Model file for the job. Use its own axes, mm. Round coordinates to 2 decimals unless told otherwise and drop trailing zeros. Order: outer loops, then holes, each group sorted by start corner. A loop starts at its lowest first (then second) coordinate and runs counter-clockwise, first axis right, second up. Notation, with made-up numbers: (24.25, 33) - (56.25, 33) arc R18 ccw to (56.25, 55) - close; hole circle Ø6 at (20, 62). An arc over 180 degrees is marked (long way). Use one line per item in the form item = value.
Autodesk Inventor part; units mm, degrees
ref_plane "Start plane" through (0, 0, 6.35) normal (0, 0, 1) x (1, 0, 0)
ref_plane "End plane" through (0, 0, 118.4911) normal (0, 0, 1) x (1, 0, 0)
ref_plane "Work Plane5" through (0, 596.3529, 6.35) normal (0, 0, -1) x (-1, 0, 0)
ref_plane "Start plane" through (0, 0, 6.35) normal (0, 0, 1) x (1, 0, 0)
ref_plane "End plane" through (0, 0, 118.4911) normal (0, 0, 1) x (1, 0, 0)
sketch "Sketch" plane through (0, 0, 0) normal (0, 0, 1) x (1, 0, 0)
  line L0 (6.35, -6.35) -> (-6.35, -6.35)
  line L1 (-6.35, -6.35) -> (-6.35, 6.35)
  line L2 (-6.35, 6.35) -> (6.35, 6.35)
  line L3 (6.35, 6.35) -> (6.35, -6.35)
  line L4 (-6, 0) -> (8, 0) construction
  line L5 (0, -30) -> (0, 40) construction
  line L6 (0, 54) -> (0, -44) construction
  line L7 (-9.62, 0) -> (13.27, 0) construction
  dimension "d0" = 12.7
  dimension "d1" = 12.7
  dimension "d4" = 6.35
  dimension "d5" = 6.35
extrude "Body" add sketch "Sketch" along normal up to surface (112.1411 mm away) from surface at 6.35
sketch "Sketch3" plane through (0, 0, 0) normal (0, 0, 1) x (1, 0, 0)
  line L0 (0, 0) -> (10, 0)
ref_plane "Work Plane3" through (0, 0, 0) normal (0, -1, 0) x (1, 0, 0)
sketch "Sketch4" plane through (0, 0, 0) normal (0, -1, 0) x (1, 0, 0)
  line L0 (-2, 6.35) -> (12, 6.35)
  line L1 (-2, 118.4911) -> (12, 118.4911)
  dimension "d9" = 112.1411
ref_plane "Work Plane5" through (0, 596.3529, 6.35) normal (0, 0, -1) x (-1, 0, 0)
split "Split2" plane through (0, 596.3529, 6.35) removes the side toward (0, 0, -1)
ref_plane "Work Plane6" through (0, -1.2326, 117.1199) normal (0, 0.2588, 0.9659) x (1, 0, 0)
split "Split3" plane through (0, -1.2326, 117.1199) removes the side toward (0, 0.2588, 0.9659)
equation "\"d0\" = G_W"
equation "\"d1\" = G_H"
equation "\"d4\" = 0.5 * d1"
equation "\"d5\" = 0.5 * d0"
equation "\"d2\" = G_L"
equation "\"G_W\" = 12.7"
equation "\"G_H\" = 12.7"
equation "\"G_L\" = d9"
equation "\"G_OFFSET_START\" = -6.35"
equation "\"G_OFFSET_END\" = -3.22903"
equation "\"d6\" = -G_OFFSET_START"
equation "\"d7\" = G_OFFSET_END + B_L"
equation "\"B_L\" = 121.72015"
properties part number "AISC - 1/2x1/2 - 4.415" material "Steel, Alloy"
(1) Slice it at B-B on y = 0.5. Give the cut face in (x, z).
Report:
outline = (-6.35, 6.35) - (6.35, 6.35) - (6.35, 116.66) - (-6.35, 116.66) - close
(2) Pin check, flat tip, straight feed: pin 1 (5 mm diameter, centred on x = -1, y = 4.5, fed in from +Z). Stop position of the tip, or through.
Report:
pin_1 = 116.25
(3) Probe probe 1 along Z at (x, y) = (-3.5, 3.25); probe 2 along Z at (x, y) = (2, 5.5). List the from-to ranges inside material, lowest first. Write a range as [from, to].
Report:
probe_1 = [6.35, 115.92]
probe_2 = [6.35, 115.32]
(4) Slice it at A-A on x = -4. Give the cut face in (y, z), then the cut area to 3 significant figures.
Report:
outline = (-6.35, 6.35) - (6.35, 6.35) - (6.35, 115.09) - (-6.35, 118.49) - close
area = 1,400 mm2
